```python
from build123d import *

# Parameters (mm, degrees)
SKETCH_W        = 60
SKETCH_H        = 50
PAD_DEPTH       = 30
SKETCH001_W     = 40
SKETCH001_H     = 30
PAD001_DEPTH    = 90
SKETCH002_W     = 35
SKETCH002_H     = 10
POCKET_DEPTH    = 50.001
SKETCH003_W     = 25
SKETCH003_H     = 26.623343
POCKET001_DEPTH = 10
SKETCH004_R     = 6
POCKET002_DEPTH = 50.001
POCKET003_DEPTH = 30.001
SKETCH006_W     = 62.083085
SKETCH006_H     = 25.997551
POCKET004_DEPTH = 10


with BuildPart() as part:
    # Sketch → Pad (new body)
    with BuildSketch(Plane.XZ):
        with Locations((0, 25)):
            Rectangle(SKETCH_W, SKETCH_H)
    extrude(amount=PAD_DEPTH)

    # Sketch001 → Pad001 (new body)
    with BuildSketch(Plane.XZ.offset(30)):
        with Locations((0, 15)):
            Rectangle(SKETCH001_W, SKETCH001_H)
    extrude(amount=PAD001_DEPTH)

    # Sketch002 → Pocket (cut, through all)
    with BuildSketch(Plane(origin=(0, 0, 50), x_dir=(-1, 0, 0), z_dir=(0, 0, 1))):
        with Locations((0, 5)):
            Rectangle(SKETCH002_W, SKETCH002_H)
    extrude(amount=-POCKET_DEPTH, mode=Mode.SUBTRACT)

    # Sketch003 → Pocket001 (cut)
    with BuildSketch(Plane(origin=(0, 0, 50), x_dir=(-1, 0, 0), z_dir=(0, 0, 1))):
        with Locations((0, 16.688329)):
            Rectangle(SKETCH003_W, SKETCH003_H)
    extrude(amount=-POCKET001_DEPTH, mode=Mode.SUBTRACT)

    # Sketch004 → Pocket002 (cut, through all)
    with BuildSketch(Plane(origin=(20, 0, 0), x_dir=(0, 0, 1), z_dir=(1, 0, 0))):
        with Locations((15, 65)):
            Circle(SKETCH004_R)
    extrude(amount=-POCKET002_DEPTH, mode=Mode.SUBTRACT)

    # Sketch005 → Pocket003 (cut, through all)
    with BuildSketch(Plane(origin=(0, 0, 30), x_dir=(-1, 0, 0), z_dir=(0, 0, 1))):
        Polygon((0, 120), (-25, 76.69873), (-25, 127.885117), (25, 127.885117), (25, 76.69873), align=None)
    extrude(amount=-POCKET003_DEPTH, mode=Mode.SUBTRACT)

    # Sketch006 → Pocket004 (cut)
    with BuildSketch(Plane(origin=(0, 0, 30), x_dir=(-1, 0, 0), z_dir=(0, 0, 1))):
        with Locations((1.302299, 112.998775)):
            Rectangle(SKETCH006_W, SKETCH006_H)
    extrude(amount=-POCKET004_DEPTH, mode=Mode.SUBTRACT)


solid = part.part
```
Model file for the job. Use its own axes, mm. A direction names the side the tool comes from. Give positions to 0.01 mm unless a question says otherwise; leave off trailing zeros. Order: outer loops, then holes, each group sorted by start corner. A loop starts at its lowest first (then second) coordinate and runs counter-clockwise, first axis right, second up.
1) Saw through at B-B, the plane y = -65. Write the cut outline in (x, z), then the cut area to 3 significant figures.
2) Saw through at D-D, the plane x = 5.5. Write the cut outline in (y, z).
3) Wall check: probe 1 along Z at (x, y) = (8, -65); probe 2 along X at (y, z) = (-8, 23.5); probe 3 along X at (y, z) = (-19, 41.5). Give the ranges that are in metal, low to high.
4) Pin check, flat tips, straight feed: pin 1 (24 mm diameter, centred on y = -46, z = 21, fed in from +X); pin 2 (3 mm diameter, centred on x = 1.5, z = 23, fed in from -Y); pin 3 (6 mm diameter, centred on x = -2.5, y = -20.5, fed in from +Z). Stop position of each tip, or through.
5) 3-axis set-ups, long thin cutter, end or side, ignore diameter. For faces 1 (the flat face through (21, -15, 50)), 2 (the flat face through (-20, -57, 15)), 3 (the flat face through (0, -10, 20)), 4 (the flat face through (12.5, -20, 45)), 5 (the flat face through (0, -100, 25)): which of +Z, -Z, +X, -X, +Y, -Y reach the whole face in a straight line?
6) Saw through at C-C, the plane z = 28.5. Write the cut outline in (x, y), then the cut area to 3 significant figures.
7) Saw through at A-A, the plane z = 15. Write the cut outline in (x, y), then the cut area to 3 significant figures.
8) Mould opens along X. For faces 6 (the flat face through (24, 0, 25)), 7 (the flat face through (-17.5, -5, 25)), 8 (the flat face through (-30, -15, 25)) say: +X half, -X half, draft (parallel to the pull), parting line (faces both ways), or undercut.
Computed:
1. outline: (-20, 0) - (20, 0) - (20, 9) - (-20, 9) - close; (-20, 21) - (20, 21) - (20, 30) - (-20, 30) - close
1. area: 720 mm2
2. outline: (-110.47, 0) - (-10, 0) - (-10, 40) - (-30, 40) - (-30, 30) - (-100, 30) - (-100, 20) - (-110.47, 20) - close; hole circle Ø12 at (-65, 15)
3. probe 1: z = 0 to 9, 21 to 30
3. probe 2: x = -30 to -17.5, 17.5 to 30
3. probe 3: x = -30 to -12.5, 12.5 to 30
4. pin 1: stops at x = 20
4. pin 2: stops at y = -100
4. pin 3: stops at z = 40
5. face 1: +Z, +X, -X, +Y, -Y
5. face 2: +Z, -Z, -X, -Y
5. face 3: +Z, -Z, +Y
5. face 4: +Z, +Y, -Y
5. face 5: +Z, +X, -X, -Y
6. outline: (-30, -30) - (-20, -30) - (-20, -85.36) - (-11.55, -100) - (11.55, -100) - (20, -85.36) - (20, -30) - (30, -30) - (30, 0) - (17.5, 0) - (17.5, -10) - (-17.5, -10) - (-17.5, 0) - (-30, 0) - close
6. area: 4,130 mm2
7. outline: (-30, -30) - (-20, -30) - (-20, -59) - (20, -59) - (20, -30) - (30, -30) - (30, 0) - (17.5, 0) - (17.5, -10) - (-17.5, -10) - (-17.5, 0) - (-30, 0) - close; (-20, -85.36) - (0, -120) - (20, -85.36) - (20, -71) - (-20, -71) - close
7. area: 3,880 mm2
8. face 6: draft
8. face 7: undercut
8. face 8: -X half
